from build123d import *

# Parameters (mm, degrees)
F0_W     = 53.975
F0_H     = 31.115
F1_DEPTH = 19.05
F2_T     = -1.5875
F3_R     = 1.5875
F4_DEPTH = 5.08
F5_W     = 12.7
F5_H     = 7.62
F6_DEPTH = 1.5875
F7_R     = 3.175


with BuildPart() as f1:
    # F0 (on Top) → F1 (new body)
    with BuildSketch(Plane.XY):
        Rectangle(F0_W, F0_H)
    extrude(amount=F1_DEPTH)

    # F2
    f2_openings = [f1.faces().sort_by_distance(p)[0] for p in [
        (0, 0, 19.05),
    ]]
    offset(amount=F2_T, openings=f2_openings)

    # F3 (on face) → F4 (join)
    with BuildSketch(Plane.XY.offset(1.5875)):
        with Locations((22.225, 10.795)):
            Circle(F3_R)
        with Locations((22.225, -10.795)):
            Circle(F3_R)
        with Locations((-22.225, 10.795)):
            Circle(F3_R)
        with Locations((-22.225, -10.795)):
            Circle(F3_R)
    extrude(amount=F4_DEPTH)

    # F5 (on face) → F6 (cut)
    with BuildSketch(Plane.YZ.offset(26.9875)):
        with Locations((0, 3.175)):
            Rectangle(F5_W, F5_H)
    extrude(amount=-F6_DEPTH, mode=Mode.SUBTRACT)

    # F7
    f7_edges = [f1.edges().sort_by_distance(p)[0] for p in [
        (26.9875, -15.5575, 9.525),
        (-26.9875, -15.5575, 9.525),
        (-26.9875, 15.5575, 9.525),
        (26.9875, 15.5575, 9.525),
    ]]
    fillet(f7_edges, radius=F7_R)


solid = f1.part
CAD build for the part. Positions are in the model's coordinates, mm. A direction names the side the tool comes from. Give positions to 0.01 mm unless a question says otherwise; leave off trailing zeros. Loops run counter-clockwise (first coordinate to the right, second up) from the corner with the lowest first, then second, coordinate; pieces in that order, holes last. Notation, with made-up numbers: M 20.25,15 L 28.25,15 A20 cw 28.25,48 Z; hole C 74.25,3.25 d1. An arc over 180 degrees is marked long. One line per question, with ' | ' between items. Start each with the question number.
1. Two-plate mould, pull along X, no slides. Class faces 4 (the face through (-22, -11, 6.668)), 5 (the face through (-26.082, -14.603, 9.658)), 6 (the face through (26, 0, 6.985)): pulls with the +X half, pulls with the -X half, needs draft (parallel to the pull), parting line crosses it, or undercut.
2. Flat gauge pins, fed straight in: pin 1 (2.5 mm diameter, centred on x = -23, y = -11, fed in from +Z); pin 2 (1.3 mm diameter, centred on x = 26, z = 4.5, fed in from +Y); pin 3 (0.8 mm diameter, centred on x = 26.5, y = 0.5, fed in from -Z) (3 decimals). Where does each tip first touch, or does it go through?
3. Saw through at C-C on y = -8.5. Give the cut face in (x, z), plus the area to 3 significant figures.
4. Saw through at D-D on z = 4.25. State how many separate pieces and enclosed holes the cut face has, plus the area to 3 significant figures.
5. Probe L1, parallel to X at y = 3, z = 10; L2, parallel to X at y = -10.5, z = 2; L3, parallel to Y at x = 10.5, z = 6.5. List the from-to ranges inside material, lowest first. Write a range as from..to.
6. 3-axis set-ups, long thin cutter, end or side, ignore diameter. For faces 1 (the face through (-22, 11, 6.668)), 2 (the face through (-26.988, 0, 9)), 3 (the face through (25.4, 0, 1)): which of +Z, -Z, +X, -X, +Y, -Y reach the whole face in a straight line?
Result sheet:
1) face 4: undercut | face 5: pulls with the -X half | face 6: needs draft
2) pin 1: stops at z = 6.67 | pin 2: stops at y = 15.16 | pin 3: stops at z = 6.985
3) outline: M -26.99,0 L 26.99,0 L 26.99,19.05 L 25.4,19.05 L 25.4,1.59 L -25.4,1.59 L -25.4,19.05 L -26.99,19.05 Z | area: 141 mm^2
4) separate pieces: 5 | enclosed holes: 0 | area: 263 mm^2
5) L1: x = -26.99..-25.4, 25.4..26.99 | L2: x = -26.99..-25.4, -23.78..-20.67, 20.67..23.78, 25.4..26.99 | L3: y = -15.56..-13.97, 13.97..15.56
6) face 1: +Z | face 2: +Z, -Z, -X, +Y, -Y | face 3: -Z, +X
